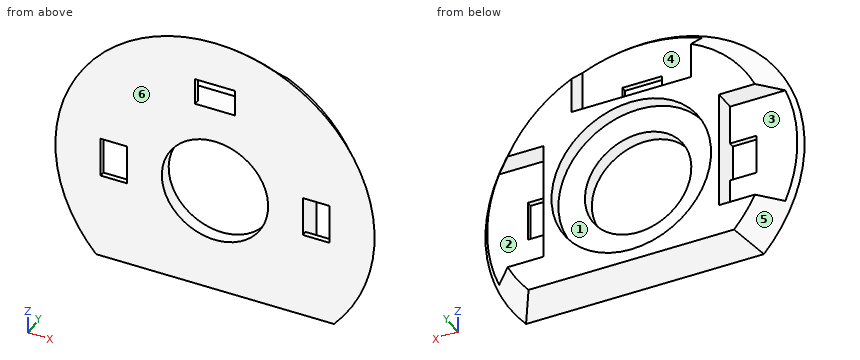
```python
from build123d import *

# Parameters (mm, degrees)
SKETCH1_R           = 60
BOSS_EXTRUDE1_DEPTH = 10
BOSS_EXTRUDE1_TAPER = 40
SKETCH2_W           = 102.123847816
SKETCH2_H           = 48.488569787
CUT_EXTRUDE1_DEPTH  = 86.440037605
CHAMFER1_SIZE2      = 5.773502692
CHAMFER1_SIZE       = 10
SKETCH3_R           = 20
CUT_EXTRUDE2_DEPTH  = 86.440037453
SKETCH4_W           = 35.035611717
SKETCH4_H           = 45
CUT_EXTRUDE3_DEPTH  = 8
SKETCH6_W           = 10
SKETCH6_H           = 15
CUT_EXTRUDE5_DEPTH  = 86.229103011
CIRPATTERN1_COUNT   = 3
CIRPATTERN1_ANGLE   = 180
SKETCH7_R           = 30
CUT_EXTRUDE6_DEPTH  = 5


with BuildPart() as part:
    # Sketch1 → Boss-Extrude1 (new body)
    with BuildSketch(Plane(origin=(0, 0, 0), x_dir=(1, 0, 0), z_dir=(0, 1, 0))):
        Circle(SKETCH1_R)
    extrude(amount=BOSS_EXTRUDE1_DEPTH, taper=BOSS_EXTRUDE1_TAPER)

    # Sketch2 → Cut-Extrude1 (cut, through all)
    with BuildSketch(Plane(origin=(0, 10, 0), x_dir=(1, 0, 0), z_dir=(0, 1, 0))):
        with Locations((-1.760755997, 64.244284894)):
            Rectangle(SKETCH2_W, SKETCH2_H)
    extrude(amount=-CUT_EXTRUDE1_DEPTH, mode=Mode.SUBTRACT)

    # Chamfer1
    chamfer1_edges = [part.edges().sort_by_distance(p)[0] for p in [
        (0, 10, -40),
    ]]
    chamfer1_side = [part.faces().sort_by_distance(p)[0] for p in [
        (0, 9.884529946, -40),
    ]]
    chamfer(chamfer1_edges, length=CHAMFER1_SIZE - 0.0001, length2=CHAMFER1_SIZE2 - 0.0001, reference=chamfer1_side[0])  # a hair under: the kernel refuses the full size

    # Sketch3 → Cut-Extrude2 (cut, through all)
    with BuildSketch(Plane(origin=(0, 10, 0), x_dir=(1, 0, 0), z_dir=(0, 1, 0))):
        with Locations(Location((0, 0, 0), (0, 0, 270))):
            Circle(SKETCH3_R)
    extrude(amount=-CUT_EXTRUDE2_DEPTH, mode=Mode.SUBTRACT)

    # Sketch4 → Cut-Extrude3 (cut)
    with BuildSketch(Plane(origin=(0, 10, 0), x_dir=(1, 0, 0), z_dir=(0, 1, 0))):
        with Locations((50.517805859, 0)):
            Rectangle(SKETCH4_W, SKETCH4_H)
    cut_extrude3 = extrude(amount=-CUT_EXTRUDE3_DEPTH, mode=Mode.SUBTRACT)

    # Sketch6 → Cut-Extrude5 (cut, through all)
    with BuildSketch(Plane(origin=(0, 2, 0), x_dir=(1, 0, 0), z_dir=(0, 1, 0))):
        with Locations((38, 0)):
            Rectangle(SKETCH6_W, SKETCH6_H)
    cut_extrude5 = extrude(amount=-CUT_EXTRUDE5_DEPTH, mode=Mode.SUBTRACT)

    # CirPattern1: Cut-Extrude3, Cut-Extrude5 ×3 about axis
    cirpattern1_axis = Axis((0, 0, 0), (0, -1, 0))
    add([cut_extrude3.rotate(cirpattern1_axis, i * CIRPATTERN1_ANGLE / (CIRPATTERN1_COUNT - 1)) for i in range(1, CIRPATTERN1_COUNT)], mode=Mode.SUBTRACT)
    add([cut_extrude5.rotate(cirpattern1_axis, i * CIRPATTERN1_ANGLE / (CIRPATTERN1_COUNT - 1)) for i in range(1, CIRPATTERN1_COUNT)], mode=Mode.SUBTRACT)

    # Sketch7 → Cut-Extrude6 (cut)
    with BuildSketch(Plane(origin=(0, 10, 0), x_dir=(1, 0, 0), z_dir=(0, 1, 0))):
        with Locations(Location((0, 0, 0), (0, 0, 270))):
            Circle(SKETCH7_R)
    extrude(amount=-CUT_EXTRUDE6_DEPTH, mode=Mode.SUBTRACT)


solid = part.part
```
Build history of the part. All positions in model axes, mm. Face numbers are marked on the shaded views. A direction names the side the tool comes from. Coordinates: 2 decimals unless noted, no trailing zeros. Order: outer loops, then holes, each group sorted by start corner. A loop starts at its lowest first (then second) coordinate and runs counter-clockwise, first axis right, second up.
Item 1: Drill centre lines: L1, parallel to X at y = 6.3, z = 0; L2, parallel to X at y = 0.5, z = 0; L3, parallel to X at y = 1.75, z = 0. Where is each one in solid material? Low to high.
Filled in:
L1: x = -33 to -30, 30 to 33
L2: x = -59.58 to -43, -33 to -20, 20 to 33, 43 to 59.58
L3: x = -58.53 to -43, -33 to -20, 20 to 33, 43 to 58.53
Item 2: Saw through at B-B on x = 0. State how many separate pieces and enclosed holes the cut face has, then the cut area to 3 significant figures.
Filled in:
separate pieces: 3
enclosed holes: 0
area: 233 mm2
Item 3: Drop flat-ended pins along their axis: pin 1 Ø6 at (x, y) = (-6.5, 4.5) entering from -Z; pin 2 Ø1.5 at (x, y) = (14.5, 5) entering from +Z; pin 3 Ø2 at (x, y) = (38.5, 0.5) entering from +Z. Give the stop position or say it passes through.
Filled in:
pin 1: stops at z = -39.13
pin 2: stops at z = 33
pin 3: stops at z = 46.73
Item 4: Saw through at C-C on y = 7.25. List the corners of the cut face in (x, z), then the cut area to 3 significant figures.
Filled in:
outline: (-49, -22.5) arc R53.92 ccw to (-40.3, -35.81) - (40.3, -35.81) arc R53.92 ccw to (49, -22.5) - (33, -22.5) - (33, 22.5) - (49, 22.5) arc R53.92 ccw to (22.5, 49) - (22.5, 33) - (-22.5, 33) - (-22.5, 49) arc R53.92 ccw to (-49, 22.5) - (-33, 22.5) - (-33, -22.5) - close; hole circle Ø60 at (0, 0)
area: 2,690 mm2
Item 5: Mould opens along X. For the marked faces 4, 5 and 6 say: released by +X, released by -X, zero draft, split by the parting line, or undercut.
Filled in:
face 4: undercut
face 5: split by the parting line
face 6: zero draft
Item 6: Saw through at A-A on z = 0. List the corners of the cut face in (x, y).
Filled in:
outline: (-60, 0) - (-43, 0) - (-43, 2) - (-58.32, 2) - close; (-33, 0) - (-20, 0) - (-20, 5) - (-30, 5) - (-30, 10) - (-33, 10) - close; (20, 0) - (33, 0) - (33, 10) - (30, 10) - (30, 5) - (20, 5) - close; (43, 0) - (60, 0) - (58.32, 2) - (43, 2) - close
Item 7: Tool access for the marked faces 1, 2 and 3: list every direction of +Z, -Z, +X, -X, +Y, -Y with a clear straight run to the whole face (end or side of a thin tool).
Filled in:
face 1: +Y
face 2: +X, +Y
face 3: -X, +Y
